from build123d import *

# Parameters (mm, degrees)
F0_W     = 42.3
F0_H     = 5
F0_R     = 8
F0_R_2   = 11
F1_DEPTH = 5
F2_DEPTH = 37
F3_DEPTH = 29


with BuildPart() as f1:
    # F0 (on Front) → F1 (new body)
    with BuildSketch(Plane.XZ):
        with Locations((0, -23.65)):
            Rectangle(F0_W, F0_H)
        Polygon((21.15, 20.15), (21.15, 1.15), (26.15, 1.15), (41.15, 1.15), (41.15, 21.15), (26.15, 21.15), (21.15, 21.15), align=None)
        with Locations((31.15, 11.15)):
            Circle(F0_R, mode=Mode.SUBTRACT)
        Polygon((21.15, 1.15), (21.15, -21.15), (21.15, -26.15), (26.15, -26.15), (26.15, 1.15), align=None)
        Polygon((-21.15, -21.15), (21.15, -21.15), (21.15, 1.15), (21.15, 20.15), (21.15, 21.15), (20.15, 21.15), (-21.15, 21.15), align=None)
        with BuildLine():
            Line((14, -15.5), (-14, -15.5))
            ThreePointArc((-14, -15.5), (-16.56066, -16.56066), (-15.5, -14))
            Line((-15.5, -14), (-15.5, 14))
            ThreePointArc((-15.5, 14), (-16.56066, 16.56066), (-14, 15.5))
            Line((-14, 15.5), (14, 15.5))
            ThreePointArc((14, 15.5), (15.5, 17), (17, 15.5))
            ThreePointArc((17, 15.5), (16.56066, 14.43934), (15.5, 14))
            Line((15.5, 14), (15.5, -14))
            ThreePointArc((15.5, -14), (16.56066, -14.43934), (17, -15.5))
            ThreePointArc((17, -15.5), (15.5, -17), (14, -15.5))
        make_face(mode=Mode.SUBTRACT)
        with BuildLine():
            ThreePointArc((-15.5, -14), (-14.43934, -14.43934), (-14, -15.5))
            Line((-14, -15.5), (14, -15.5))
            ThreePointArc((14, -15.5), (14.43934, -14.43934), (15.5, -14))
            Line((15.5, -14), (15.5, 14))
            ThreePointArc((15.5, 14), (14.43934, 14.43934), (14, 15.5))
            Line((14, 15.5), (-14, 15.5))
            ThreePointArc((-14, 15.5), (-14.43934, 14.43934), (-15.5, 14))
            Line((-15.5, 14), (-15.5, -14))
        make_face()
        Circle(F0_R_2, mode=Mode.SUBTRACT)
    extrude(amount=-F1_DEPTH)

    # F0 (on Front) → F2 (join)
    with BuildSketch(Plane.XZ):
        with Locations((0, -23.65)):
            Rectangle(F0_W, F0_H)
        Polygon((21.15, 1.15), (21.15, -21.15), (21.15, -26.15), (26.15, -26.15), (26.15, 1.15), align=None)
    extrude(amount=-F2_DEPTH)

    # F0 (on Front) → F3 (join)
    with BuildSketch(Plane.XZ):
        Polygon((21.15, 20.15), (21.15, 1.15), (26.15, 1.15), (41.15, 1.15), (41.15, 21.15), (26.15, 21.15), (21.15, 21.15), align=None)
        with Locations((31.15, 11.15)):
            Circle(F0_R, mode=Mode.SUBTRACT)
    extrude(amount=-F3_DEPTH)


solid = f1.part
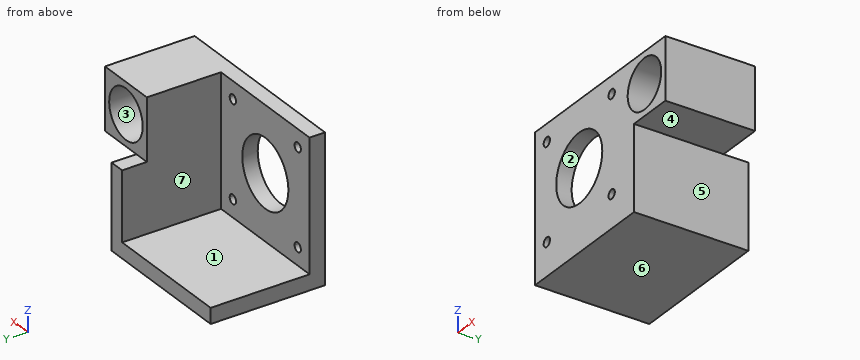
Could you check a few things on this model? Use its own coordinates, in mm. Face numbers are marked on the shaded views. A direction names the side the tool comes from. Round coordinates to 2 decimals unless told otherwise and drop trailing zeros. Loops run counter-clockwise (first coordinate to the right, second up) from the corner with the lowest first, then second, coordinate; pieces in that order, holes last. Notation, with made-up numbers: (47.25, 42.5) - (95.25, 42.5) arc R33 cw to (95.25, 77.5) - close; hole circle Ø11 at (29.5, 72). An arc over 180 degrees is marked (long way). Write item = value, one per line.
1) I'm going to push flat-ended pins straight in: P1, Ø5, axis at y = 27, z = -1.5, coming from the +X side; P2, Ø12, axis at x = 36.5, y = 19, coming from the -Z side; P3, Ø12.5, axis at x = 9, z = -3.5, coming from the +Y side. Where does each tip first touch, or does it pass through?
Computed:
P1 = 26.15
P2 = 1.15
P3 = 5
2) On a 3-axis mill with a long thin cutter (end or side, diameter ignored), from which of +Z, -Z, +X, -X, +Y, -Y can I reach the whole of each face in a straight line? I mean the marked faces 5, 6 and 7. Say none if no direction works.
Computed:
face_5 = -Z, +X, +Y, -Y
face_6 = -Z, +X, -X, +Y, -Y
face_7 = +Z, -X, +Y
3) Imagine slicing it at D-D (y = 31). Please give me the cut outline in (x, z).
Computed:
outline = (-21.15, -26.15) - (26.15, -26.15) - (26.15, 1.15) - (21.15, 1.15) - (21.15, -21.15) - (-21.15, -21.15) - close
4) Imagine slicing it at B-B (y = 14). Please give me the cut outline in (x, z), and give its area (3 significant figures).
Computed:
outline = (-21.15, -26.15) - (26.15, -26.15) - (26.15, 1.15) - (41.15, 1.15) - (41.15, 21.15) - (21.15, 21.15) - (21.15, -21.15) - (-21.15, -21.15) - close; hole circle Ø16 at (31.15, 11.15)
area = 547 mm2
5) If we mould it in two halves opening along Z, with no side actions, what happens to the marked faces 1, 2, 3 and 4? For each: pulls with the +Z half, pulls with the -Z half, needs draft (parallel to the pull), parting line crosses it, or undercut.
Computed:
face_1 = pulls with the +Z half
face_2 = undercut
face_3 = undercut
face_4 = pulls with the -Z half
6) Imagine slicing it at A-A (x = 31.15). Please give me the cut outline in (y, z), and give its area (3 significant figures).
Computed:
outline = (0, 1.15) - (29, 1.15) - (29, 3.15) - (0, 3.15) - close; (0, 19.15) - (29, 19.15) - (29, 21.15) - (0, 21.15) - close
area = 116 mm2
7) Imagine slicing it at C-C (z = -3). Please give me the cut outline in (x, y).
Computed:
outline = (-21.15, 0) - (-10.58, 0) - (-10.58, 5) - (-21.15, 5) - close; (10.58, 0) - (26.15, 0) - (26.15, 37) - (21.15, 37) - (21.15, 5) - (10.58, 5) - close
8) I need wall thicknesses on line 1 along X through (y, z) = (3.4, -15.5); line 2 along Z through (x, y) = (-15.5, 3.5); line 3 along Z through (x, y) = (0, 3). Which ranges of each line are inside material? Lowest first, please. Write a range as from..to.
Computed:
line_1 = -21.15..-17, -14..14, 17..26.15
line_2 = -26.15..-17, -14..14, 17..21.15
line_3 = -26.15..-11, 11..21.15
